Part model, mm, in its own coordinate system. A direction names the side the tool comes from. Give positions to 0.01 mm unless a question says otherwise; leave off trailing zeros. Order: outer loops, then holes, each group sorted by start corner. A loop starts at its lowest first (then second) coordinate and runs counter-clockwise, first axis right, second up. Notation, with made-up numbers: M 29,83 L 53,83 A11 ccw 53,100 Z; hole C 19,77.5 d5. An arc over 180 degrees is marked long. Answer as a JSON object with one key per item and string values.
from build123d import *

# Parameters (mm, degrees)
EXTRUDE_1_DEPTH = 12
FILLET_1_R      = 5


with BuildPart() as part:
    # 草图1 → 凸台-拉伸1 (new body)
    with BuildSketch(Plane.XY):
        with BuildLine():
            Line((-16, -8), (-10, -8))
            Line((-10, -8), (-10, 0))
            ThreePointArc((-10, 0), (0, 10), (10, 0))
            Line((10, 0), (10, -16))
            Line((10, -16), (16, -16))
            Line((16, -16), (16, 0))
            ThreePointArc((16, 0), (0, 16), (-16, 0))
            Line((-16, 0), (-16, -8))
        make_face()
        Polygon((16, -16), (10, -16), (-10, -16), (-16, -16), (-22, -16), (-22, -54), (-16, -54), (-16, -22), (-10, -22), (10, -22), (16, -22), (16, -54), (22, -54), (22, -16), align=None)
        Polygon((16, -54), (22, -54), (22, -60.12975141), (-22, -60.12975141), (-22, -54), (-16, -54), align=None)
    extrude(amount=EXTRUDE_1_DEPTH)

    # 圆角1
    fillet_1_edges = [part.edges().sort_by_distance(p)[0] for p in [
        (16, -16, 6),
    ]]
    fillet(fillet_1_edges, radius=FILLET_1_R)


solid = part.part
1. Cut at A-A on x = 0. Give the cut face in (y, z).
Worked answers:
{"outline": "M -60.13,0 L -54,0 L -54,12 L -60.13,12 Z; M -22,0 L -16,0 L -16,12 L -22,12 Z; M 10,0 L 16,0 L 16,12 L 10,12 Z"}
2. Cut at B-B on y = -39.5. Give the cut face in (x, z).
Worked answers:
{"outline": "M -22,0 L -16,0 L -16,12 L -22,12 Z; M 16,0 L 22,0 L 22,12 L 16,12 Z"}
3. Cut at D-D on x = 13. Give the cut face in (y, z), plus the area to 3 significant figures.
Worked answers:
{"outline": "M -60.13,0 L -54,0 L -54,12 L -60.13,12 Z; M -22,0 L 9.33,0 L 9.33,12 L -22,12 Z", "area": "449 mm^2"}
4. Two-plate mould, pull along X, no slides. Class faces 1 (the flat face through (-0.3, -21.5, 0)), 2 (the flat face through (-16, -38, 6)), 3 (the flat face through (16, -6, 6)): +X half, -X half, draft (parallel to the pull), parting line (faces both ways), or undercut.
Worked answers:
{"face 1": "draft", "face 2": "undercut", "face 3": "+X half"}
5. Cut at C-C on z = 10.25. Give the cut face in (x, y).
Worked answers:
{"outline": "M -22,-60.13 L 22,-60.13 L 22,-16 L 21,-16 A5 cw 16,-11 L 16,0 A16 ccw -16,0 L -16,-8 L -10,-8 L -10,0 A10 cw 10,0 L 10,-16 L -22,-16 Z; hole M -16,-54 L 16,-54 L 16,-22 L -16,-22 Z"}
6. Which spindle directions (+Z, -Z, +X, -X, +Y, -Y) get a long thin tool onto all of the face, cutting with end or side? Do faces 4 (the flat face through (10, -8, 6)), 5 (the flat face through (-16, -4, 6)), 6 (the flat face through (-6, -16, 6)), 7 (the flat face through (-22, -38, 6)), 8 (the flat face through (-0.3, -21.5, 12)). Say none if no direction does.
Worked answers:
{"face 4": "+Z, -Z", "face 5": "+Z, -Z, -X, +Y", "face 6": "+Z, -Z, -X", "face 7": "+Z, -Z, -X, +Y, -Y", "face 8": "+Z, +X, -X, +Y, -Y"}
7. Probe line 1 along X through (y, z) = (-3.5, 9.25); line 2 along X through (y, z) = (-33.5, 5); line 3 along Y through (x, z) = (2, 7.25). List the from-to ranges inside material, lowest first.
Worked answers:
{"line 1": "x = -16 to -10, 10 to 16", "line 2": "x = -22 to -16, 16 to 22", "line 3": "y = -60.13 to -54, -22 to -16, 9.8 to 15.87"}
8. Pin check, flat tips, straight feed: P1, Ø3.5, axis at y = -11, z = 4.5, coming from the -X side; P2, Ø4, axis at y = -3.5, z = 8, coming from the +X side; P3, Ø2.5, axis at y = -4, z = 4, coming from the -X side. Stop position of each tip, or through.
Worked answers:
{"P1": "stops at x = 10", "P2": "stops at x = 16", "P3": "stops at x = -16"}
